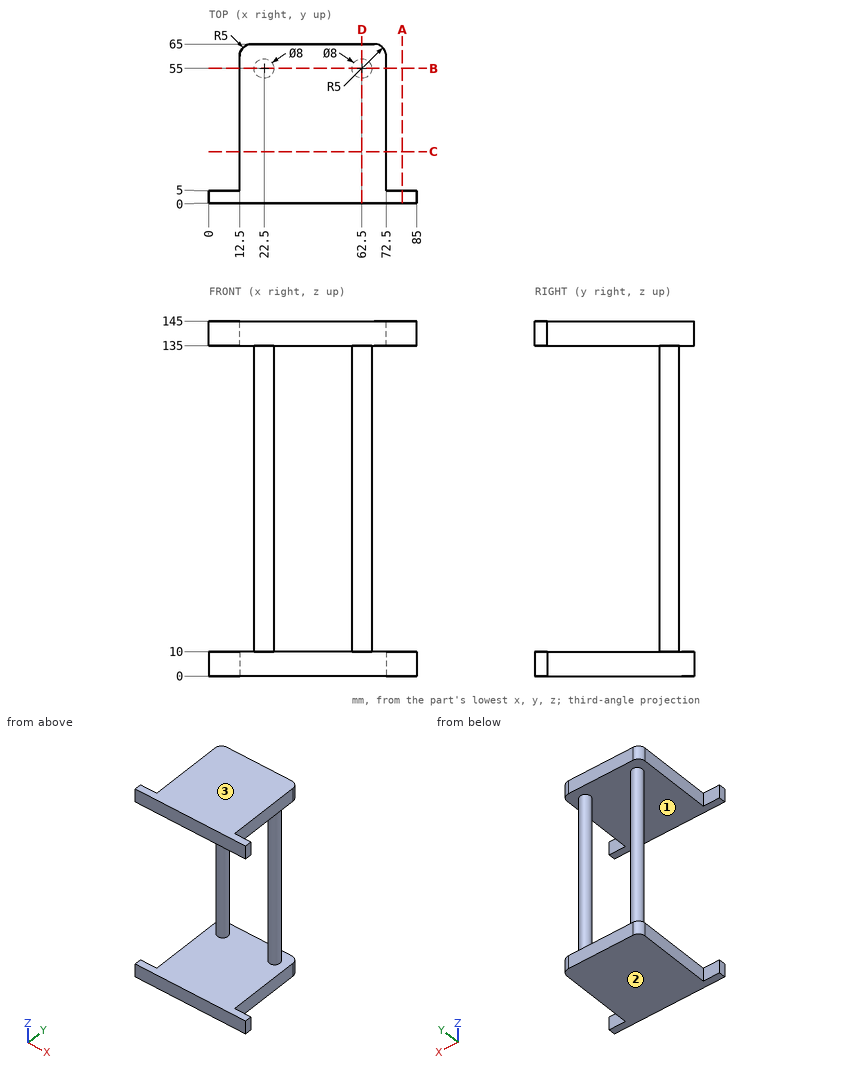
Drawing for the job (mm, zero at the part's lowest x, y, z). Coordinates: 2 decimals unless noted, no trailing zeros. Order: outer loops, then holes, each group sorted by start corner. A loop starts at its lowest first (then second) coordinate and runs counter-clockwise, first axis right, second up.
Item 1: Band-saw the part on D-D on x = 62.5. List the corners of the cut face in (y, z), plus the area to 3 significant figures.
Check sheet entries:
outline: (0, 0) - (65, 0) - (65, 10) - (59, 10) - (59, 135) - (65, 135) - (65, 145) - (0, 145) - (0, 135) - (51, 135) - (51, 10) - (0, 10) - close
area: 2,300 mm2
Item 2: Band-saw the part on C-C on y = 21. List the corners of the cut face in (x, z), plus the area to 3 significant figures.
Check sheet entries:
outline: (12.5, 0) - (72.5, 0) - (72.5, 10) - (12.5, 10) - close; (12.5, 135) - (72.5, 135) - (72.5, 145) - (12.5, 145) - close
area: 1,200 mm2
Item 3: Pin check, flat tips, straight feed: pin 1 Ø5 at (x, z) = (76.5, 138.5) entering from +Y; pin 2 Ø5 at (y, z) = (43.5, 139) entering from -X; pin 3 Ø11 at (y, z) = (25, 138.5) entering from +X. Stop position of each tip, or through.
Check sheet entries:
pin 1: stops at y = 5
pin 2: stops at x = 12.5
pin 3: stops at x = 72.5
Item 4: Two-plate mould, pull along Z, no slides. Class the marked faces 1, 2 and 3: +Z half, -Z half, draft (parallel to the pull), parting line (faces both ways), or undercut.
Check sheet entries:
face 1: undercut
face 2: -Z half
face 3: +Z half
Item 5: Band-saw the part on A-A on x = 79. List the corners of the cut face in (y, z).
Check sheet entries:
outline: (0, 0) - (5, 0) - (5, 10) - (0, 10) - close; (0, 135) - (5, 135) - (5, 145) - (0, 145) - close
Item 6: Drill centre lines: L1, parallel to Z at x = 66.5, y = 57; L2, parallel to X at y = 53.5, z = 63; L3, parallel to X at y = 57, z = 101.5. Where is each one in solid material? Low to high.
Check sheet entries:
L1: z = 0 to 10, 135 to 145
L2: x = 18.79 to 26.21, 58.79 to 66.21
L3: x = 19.04 to 25.96, 59.04 to 65.96
Item 7: Band-saw the part on B-B on y = 55. List the corners of the cut face in (x, z), plus the area to 3 significant figures.
Check sheet entries:
outline: (12.5, 0) - (72.5, 0) - (72.5, 10) - (66.5, 10) - (66.5, 135) - (72.5, 135) - (72.5, 145) - (12.5, 145) - (12.5, 135) - (18.5, 135) - (18.5, 10) - (12.5, 10) - close; hole (26.5, 10) - (58.5, 10) - (58.5, 135) - (26.5, 135) - close
area: 3,200 mm2
